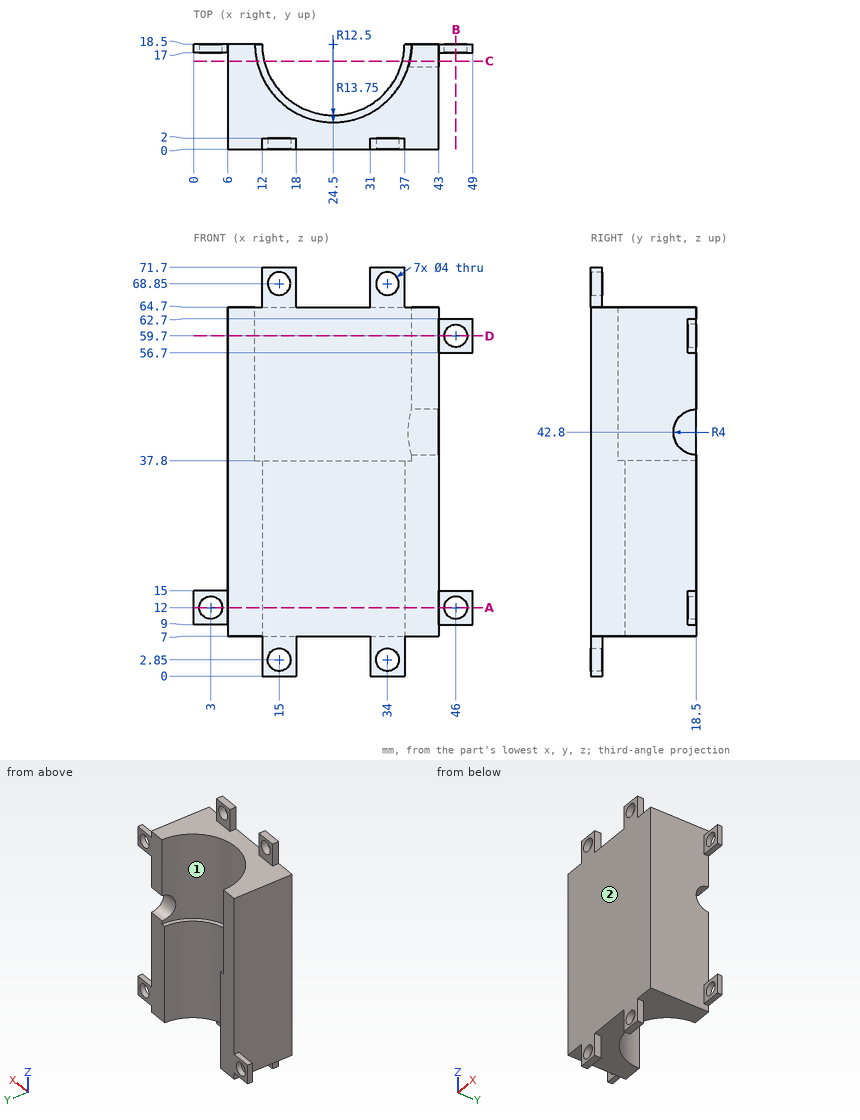
Answer from the drawing. Dimensions are ordinates in mm from the lowest x, y and z of the part. A direction names the side the tool comes from. Round coordinates to 2 decimals unless told otherwise and drop trailing zeros. Write each loop counter-clockwise with the first axis right and the second up, starting at its lowest first coordinate (ties: lowest second). Pieces come first, ordered by that corner, then holes. Notation, with made-up numbers: M -29,-1 L -25,-1 A25 ccw -25,16 Z; hole C 44,49.25 d11. An arc over 180 degrees is marked long. One line per item, written item: value.
Q1. Find section D-D on z = 59.7. Write down the section's boundary in (x, y).
Data:
outline: M 6,0 L 43,0 L 43,17 L 44,17 L 44,18.5 L 38.25,18.5 A13.75 cw 10.75,18.5 L 6,18.5 Z; M 48,17 L 49,17 L 49,18.5 L 48,18.5 Z
Q2. Find section B-B on x = 46. Write down the section's boundary in (y, z), plus the area to 3 significant figures.
Data:
outline: M 17,9 L 18.5,9 L 18.5,10 L 17,10 Z; M 17,14 L 18.5,14 L 18.5,15 L 17,15 Z; M 17,56.7 L 18.5,56.7 L 18.5,57.7 L 17,57.7 Z; M 17,61.7 L 18.5,61.7 L 18.5,62.7 L 17,62.7 Z
area: 6.00 mm2
Q3. Flat-ended cylindrical pins translate along their axes: pin 1 Ø1.2 at (x, y) = (46, 17.5) entering from -Z; pin 2 Ø1 at (y, z) = (1, 67.5) entering from +X; pin 3 Ø4.5 at (x, z) = (46, 59.7) entering from -Y. Find the tip coordinate at first contact, or state that the pin passes through.
Data:
pin 1: z = 9
pin 2: x = 37
pin 3: y = 17
Q4. Find section A-A on z = 12. Write down the section's boundary in (x, y), plus the area to 3 significant figures.
Data:
outline: M 0,17 L 1,17 L 1,18.5 L 0,18.5 Z; M 5,17 L 6,17 L 6,0 L 43,0 L 43,17 L 44,17 L 44,18.5 L 37,18.5 A12.5 cw 12,18.5 L 5,18.5 Z; M 48,17 L 49,17 L 49,18.5 L 48,18.5 Z
area: 445 mm2
Q5. Which of the six approach directions +Z, -Z, +X, -X, +Y, -Y give full straight-line access (tool end or side, diameter ignored) to the marked faces 1 and 2?
Data:
face 1: +Z, +Y
face 2: +Z, -Z, +X, -X, -Y
Q6. Find section C-C on y = 15.5. Write down the section's boundary in (x, z).
Data:
outline: M 6,7 L 12.37,7 L 12.37,37.8 L 11.08,37.8 L 11.08,64.7 L 6,64.7 Z; M 36.63,7 L 43,7 L 43,40.15 L 37.92,40.15 L 37.92,37.8 L 36.63,37.8 Z; M 37.92,45.45 L 43,45.45 L 43,64.7 L 37.92,64.7 Z
Q7. Straight lines are drawn through the part: line 1 (X direction, y = 0.55, z = 68.85); line 2 (X direction, y = 17.8, z = 59.7); line 3 (X direction, y = 11, z = 39). For each, find the intervals that lie inside material, in ascending order. Write a range as [from, to].
Data:
line 1: [12, 13], [17, 18], [31, 32], [36, 37]
line 2: [6, 10.77], [38.23, 44], [48, 49]
line 3: [6, 12.98], [36.02, 43]
